Input: part model. Units: mm. Frame: model coordinates. Face numbers are marked on the shaded views. A direction names the side the tool comes from. Coordinates: 2 decimals unless noted, no trailing zeros. Order: outer loops, then holes, each group sorted by start corner. A loop starts at its lowest first (then second) coordinate and runs counter-clockwise, first axis right, second up. Notation, with made-up numbers: M -21,-7 L -9,-7 A20 ccw -9,16 Z; hole C -11,-14 d9. An arc over 180 degrees is marked long. Answer in a Markdown table with one row per item.
from build123d import *

# Parameters (mm, degrees)
F0_R     = 38.1
F1_DEPTH = 23.8125
F2_W     = 57.15
F2_H     = 16.66875
F3_DEPTH = 21.43125
F5_DEPTH = 25.4
F6_R     = 2.54
F6_W     = 1.9685
F6_H     = 12.000408
F7_DEPTH = 25.4
F8_R     = 1.27


with BuildPart() as f1:
    # F0 (on Front) → F1 (new body)
    with BuildSketch(Plane.XZ):
        Circle(F0_R)
    extrude(amount=F1_DEPTH)

    # F2 (on face) → F3 (cut)
    with BuildSketch(Plane.XZ.offset(23.8125)):
        with Locations((0, 10.31875)):
            Rectangle(F2_W, F2_H)
        with Locations((0, -10.31875)):
            Rectangle(F2_W, F2_H)
    extrude(amount=-F3_DEPTH, mode=Mode.SUBTRACT)

    # F4 (on face) → F5 (cut)
    with BuildSketch(Plane.XZ.offset(23.8125)):
        with BuildLine():
            Line((-30.48, 22.86), (30.48, 22.86))
            ThreePointArc((30.48, 22.86), (0, 38.1), (-30.48, 22.86))
        make_face()
        with BuildLine():
            ThreePointArc((-30.48, -22.86), (0, -38.1), (30.48, -22.86))
            Line((30.48, -22.86), (-30.48, -22.86))
        make_face()
    extrude(amount=-F5_DEPTH, mode=Mode.SUBTRACT)

    # F6 (on face) → F7 (cut, symmetric)
    with BuildSketch(Plane.XZ.offset(2.38125)):
        with Locations((21.43125, -10.31875)):
            Circle(F6_R)
        Polygon((18.89125, 9.04875), (23.97125, 9.04875), (23.97125, 11.58875), (22.00275, 11.58875), (18.89125, 11.58875), align=None)
        with Locations((22.987, 17.588954)):
            Rectangle(F6_W, F6_H)
    extrude(amount=F7_DEPTH, both=True, mode=Mode.SUBTRACT)

    # F8
    f8_edges = [f1.edges().sort_by_distance(p)[0] for p in [
        (23.97125, -23.8125, 20.756562),
        (22.00275, -23.8125, 20.756562),
    ]]
    fillet(f8_edges, radius=F8_R)


solid = f1.part
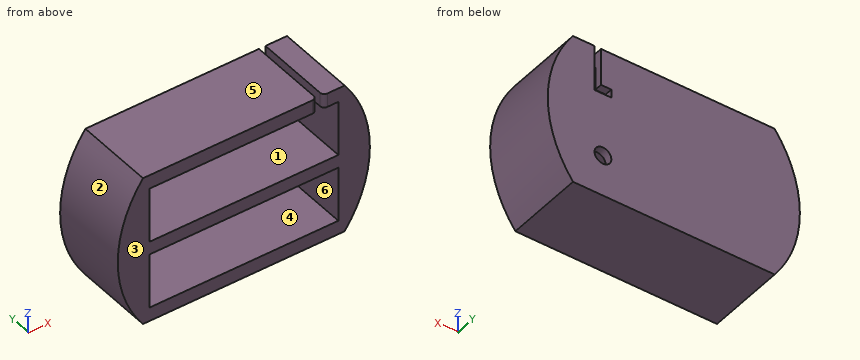
1) Cut plane C-C, the plane z = 16. Output: boundary loops of the cut face in (x, y) (1 decimal).
Resolved:
| item | result |
|---|---|
| outline | M -34.6,-23.8 L -28.6,-23.8 L -28.6,-2.4 L 22,-2.4 L 22,0 L -34.6,0 Z; M 24,-2.4 L 28.6,-2.4 L 28.6,-23.8 L 34.6,-23.8 L 34.6,0 L 24,0 Z |
2) Reachability of the marked faces 5 and 6 from +Z, -Z, +X, -X, +Y, -Y: full face, straight path, thin tool, end or side. Return the list, or none.
Resolved:
| item | result |
|---|---|
| face 5 | +Z, +X, -X, +Y, -Y |
| face 6 | -Y |
3) Cut plane D-D, the plane z = 4. Output: boundary loops of the cut face in (x, y) (1 decimal), and give its area (3 significant figures).
Resolved:
| item | result |
|---|---|
| outline | M -37.9,-23.8 L -28.6,-23.8 L -28.6,-2.4 L 28.6,-2.4 L 28.6,-23.8 L 37.9,-23.8 L 37.9,0 L -37.9,0 Z |
| area | 580 mm2 |
4) Contact query for flat-ended pins moving along their axis: pin 1 (8.5 mm diameter, centred on y = -18, z = -12, fed in from -X); pin 2 (1.2 mm diameter, centred on y = -1, z = 10, fed in from +X); pin 3 (7 mm diameter, centred on y = -11.5, z = 16.5, fed in from -X); pin 4 (3 mm diameter, centred on x = 21.43, z = -10.32, fed in from +Y). Output: stop coordinate, or through.
Resolved:
| item | result |
|---|---|
| pin 1 | stops at x = -37.3 |
| pin 2 | stops at x = 36.92 |
| pin 3 | stops at x = -35.81 |
| pin 4 | passes through |
5) Mould query, pull axis X, two halves, no side actions, for the marked faces 1, 2, 3 and 4. Classes: +X half, -X half, draft (parallel to the pull), parting line (faces both ways), or undercut.
Resolved:
| item | result |
|---|---|
| face 1 | undercut |
| face 2 | -X half |
| face 3 | draft |
| face 4 | undercut |
6) Material intervals for probe 1 along Z at (x, y) = (9, -14.75); probe 2 along Z at (x, y) = (23.5, -4); probe 3 along X at (y, z) = (-22.5, 0), sorted ascending.
Resolved:
| item | result |
|---|---|
| probe 1 | z = -22.86 to -18.65, -1.98 to 1.98, 18.65 to 22.86 |
| probe 2 | z = -22.86 to -18.65, -1.98 to 1.98 |
| probe 3 | x = -38.1 to 38.1 |
7) Cut plane B-B, the plane x = 26.5. Output: boundary loops of the cut face in (y, z).
Resolved:
| item | result |
|---|---|
| outline | M -23.81,-22.86 L 0,-22.86 L 0,22.86 L -23.81,22.86 L -23.81,18.65 L -2.38,18.65 L -2.38,1.98 L -23.81,1.98 L -23.81,-1.98 L -2.38,-1.98 L -2.38,-18.65 L -23.81,-18.65 Z |
8) Cut plane A-A, the plane y = -12.5. Output: boundary loops of the cut face in (x, z) (3 decimals), and give its area (3 significant figures).
Resolved:
| item | result |
|---|---|
| outline | M -30.48,-22.86 L 30.48,-22.86 A38.1 ccw 30.48,22.86 L 23.971,22.86 L 23.971,18.653 L 28.575,18.653 L 28.575,1.984 L -28.575,1.984 L -28.575,18.653 L 22.003,18.653 L 22.003,22.86 L -30.48,22.86 A38.1 ccw Z; hole M -28.575,-18.653 L 28.575,-18.653 L 28.575,-1.984 L -28.575,-1.984 Z |
| area | 1,350 mm2 |
